```python
from build123d import *

# Parameters (mm, degrees)
F3_W      = 16
F3_H      = 16
F6_DEPTH  = 40
F4_W      = 16
F4_H      = 16
F7_DEPTH  = 40
F5_W      = 16
F5_H      = 16
F8_DEPTH  = 40
F9_D      = 2.5
F9_DEPTH  = 13
F9_TIP    = 0.7510757738
F10_D     = 4
F10_DEPTH = 2
F10_TIP   = 1.2017212381
F11_D     = 2.5
F11_DEPTH = 13
F11_TIP   = 0.7510757738
F12_D     = 4
F12_DEPTH = 2
F12_TIP   = 1.2017212381
F13_D     = 2.5
F13_DEPTH = 13
F13_TIP   = 0.7510757738
F14_D     = 4
F14_DEPTH = 2
F14_TIP   = 1.2017212381


with BuildPart() as f6:
    # F3 (on offset) → F6 (new body)
    with BuildSketch(Plane.XZ.offset(17.5)):
        with Locations((-9.5, -9.5)):
            Rectangle(F3_W, F3_H)
    extrude(amount=-F6_DEPTH)

    # F4 (on offset) → F7 (join)
    with BuildSketch(Plane.YZ.offset(-17.5)):
        with Locations((-9.5, -9.5)):
            Rectangle(F4_W, F4_H)
    extrude(amount=F7_DEPTH)

    # F5 (on offset) → F8 (join)
    with BuildSketch(Plane.XY.offset(-17.5)):
        with Locations((-9.5, -9.5)):
            Rectangle(F5_W, F5_H)
    extrude(amount=F8_DEPTH)

    # F9
    with Locations(Plane(origin=(0, 0, -17.5), x_dir=(1, 0, 0), z_dir=(0, 0, -1))):
        with Locations((6, 9.5)):
            Hole(F9_D / 2, depth=F9_DEPTH)
            with Locations((0, 0, -(F9_DEPTH + F9_TIP / 2))):  # 118° drill point
                Cone(0, F9_D / 2, F9_TIP, mode=Mode.SUBTRACT)

    # F10
    with Locations(Plane(origin=(0, 0, -17.5), x_dir=(1, 0, 0), z_dir=(0, 0, -1))):
        with Locations((6, 9.5)):
            Hole(F10_D / 2, depth=F10_DEPTH)
            with Locations((0, 0, -(F10_DEPTH + F10_TIP / 2))):  # 118° drill point
                Cone(0, F10_D / 2, F10_TIP, mode=Mode.SUBTRACT)

    # F11
    with Locations(Plane(origin=(0, 0, -17.5), x_dir=(1, 0, 0), z_dir=(0, 0, -1))):
        with Locations((-9.5, -6)):
            Hole(F11_D / 2, depth=F11_DEPTH)
            with Locations((0, 0, -(F11_DEPTH + F11_TIP / 2))):  # 118° drill point
                Cone(0, F11_D / 2, F11_TIP, mode=Mode.SUBTRACT)

    # F12
    with Locations(Plane(origin=(0, 0, -17.5), x_dir=(1, 0, 0), z_dir=(0, 0, -1))):
        with Locations((-9.5, -6)):
            Hole(F12_D / 2, depth=F12_DEPTH)
            with Locations((0, 0, -(F12_DEPTH + F12_TIP / 2))):  # 118° drill point
                Cone(0, F12_D / 2, F12_TIP, mode=Mode.SUBTRACT)

    # F13
    with Locations(Plane(origin=(-17.5, 0, 0), x_dir=(0, 1, 0), z_dir=(-1, 0, 0))):
        with Locations((-9.5, -6)):
            Hole(F13_D / 2, depth=F13_DEPTH)
            with Locations((0, 0, -(F13_DEPTH + F13_TIP / 2))):  # 118° drill point
                Cone(0, F13_D / 2, F13_TIP, mode=Mode.SUBTRACT)

    # F14
    with Locations(Plane(origin=(-17.5, 0, 0), x_dir=(0, 1, 0), z_dir=(-1, 0, 0))):
        with Locations((-9.5, -6)):
            Hole(F14_D / 2, depth=F14_DEPTH)
            with Locations((0, 0, -(F14_DEPTH + F14_TIP / 2))):  # 118° drill point
                Cone(0, F14_D / 2, F14_TIP, mode=Mode.SUBTRACT)


solid = f6.part
```
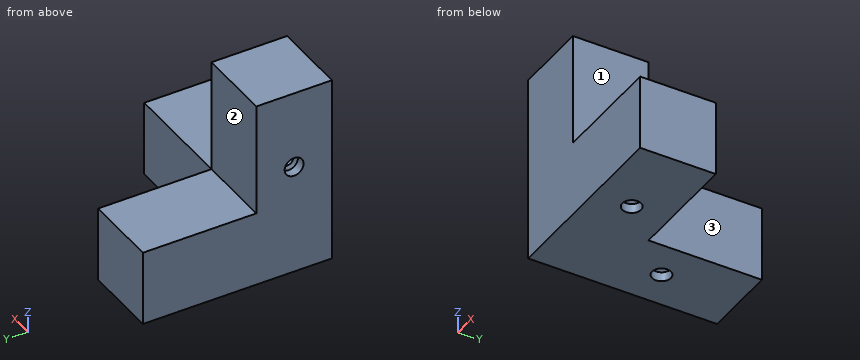
Geometry: final body of the model. Coordinates: model frame, mm. Face numbers are marked on the shaded views. A direction names the side the tool comes from. Round coordinates to 2 decimals unless told otherwise and drop trailing zeros. Write each loop counter-clockwise with the first axis right and the second up, starting at its lowest first coordinate (ties: lowest second). Pieces come first, ordered by that corner, then holes. Notation, with made-up numbers: M 64.25,33.25 L 71.25,33.25 A23 cw 71.25,60.25 Z; hole C 20,47 d2. An arc over 180 degrees is marked long. Answer in a Markdown table with one row per item. Add a question column.
(1) Ray query, L1, parallel to Z at x = -16.2, y = -9.5; L2, parallel to Y at x = -9.5, z = -11.5. Return the intervals inside material, ascending.
(2) Cut plane B-B, the plane y = -13. Return the cut outline in (x, z).
(3) Cut plane C-C, the plane z = 11. Return the cut outline in (x, y), then the cut area to 3 significant figures.
(4) Reachability of the marked faces 1, 2 and 3 from +Z, -Z, +X, -X, +Y, -Y: full face, straight path, thin tool, end or side. Return the list, or none.
(5) Contact query for flat-ended pins moving along their axis: pin 1 (1.5 mm diameter, centred on x = -9.5, y = 6, fed in from +Z); pin 2 (5 mm diameter, centred on x = -6.5, z = 16.5, fed in from +Y); pin 3 (1.5 mm diameter, centred on y = -9.5, z = 6, fed in from -X). Output: stop coordinate, or through.
(6) Cut plane A-A, the plane x = -6. Return the cut outline in (y, z), then the cut area to 3 significant figures.
Established:
| question | item | result |
|---|---|---|
| 1 | L1 | -17.5 to 4, 8 to 22.5 |
| 1 | L2 | -17.5 to 4.75, 7.25 to 22.5 |
| 2 | outline | M -17.5,-17.5 L 22.5,-17.5 L 22.5,-1.5 L -1.5,-1.5 L -1.5,22.5 L -17.5,22.5 Z |
| 3 | outline | M -17.5,-17.5 L -1.5,-17.5 L -1.5,-1.5 L -17.5,-1.5 Z |
| 3 | area | 256 mm² |
| 4 | face 1 | +Z, +X, +Y, -Y |
| 4 | face 2 | +Z, +X, -X, +Y |
| 4 | face 3 | +Z, -Z, +X, +Y |
| 5 | pin 1 | z = -1.5 |
| 5 | pin 2 | y = -1.5 |
| 5 | pin 3 | x = -4.2 |
| 6 | outline | M -17.5,-17.5 L 22.5,-17.5 L 22.5,-1.5 L -1.5,-1.5 L -1.5,22.5 L -17.5,22.5 Z; hole C -9.5,6 d2.5 |
| 6 | area | 1,020 mm² |
